CAD build for the part. Positions are in the model's coordinates, mm. A direction names the side the tool comes from. Coordinates: 2 decimals unless noted, no trailing zeros. Loops run counter-clockwise (first coordinate to the right, second up) from the corner with the lowest first, then second, coordinate; pieces in that order, holes last. Notation, with made-up numbers: (88.5, 13.5) -> (134.5, 13.5) arc R30 ccw to (134.5, 52.5) -> close; hole circle Ø10 at (-19.75, 32.5). An arc over 180 degrees is marked (long way). Answer as CSV lines item,"result". Start each with the question number.
from build123d import *

# Parameters (mm, degrees)
SKETCH2_W           = 120
SKETCH2_H           = 55
BOSS_EXTRUDE1_DEPTH = 20
SKETCH3_W           = 20
SKETCH3_H           = 35
CUT_EXTRUDE1_DEPTH  = 20
BOSS_EXTRUDE2_DEPTH = 10


with BuildPart() as part:
    # Sketch2 → Boss-Extrude1 (new body)
    with BuildSketch(Plane(origin=(0, 0, 0), x_dir=(1, 0, 0), z_dir=(0, 1, 0))):
        Rectangle(SKETCH2_W, SKETCH2_H)
    extrude(amount=BOSS_EXTRUDE1_DEPTH)

    # Sketch3 → Cut-Extrude1 (cut)
    with BuildSketch(Plane(origin=(0, 0, 0), x_dir=(-1, 0, 0), z_dir=(0, -1, 0))):
        with Locations((40, 0)):
            Rectangle(SKETCH3_W, SKETCH3_H)
        with Locations((-40, 0)):
            Rectangle(SKETCH3_W, SKETCH3_H)
    extrude(amount=-CUT_EXTRUDE1_DEPTH, mode=Mode.SUBTRACT)

    # Sketch4 → Boss-Extrude2 (add)
    with BuildSketch(Plane(origin=(0, 20, 0), x_dir=(1, 0, 0), z_dir=(0, 1, 0))):
        with BuildLine():
            ThreePointArc((-60, 27.5), (-87.5, 0), (-60, -27.5))
            Line((-60, -27.5), (-60, 27.5))
        make_face()
        with BuildLine():
            ThreePointArc((60, 27.5), (87.5, 0), (60, -27.5))
            Line((60, -27.5), (60, 27.5))
        make_face()
    extrude(amount=-BOSS_EXTRUDE2_DEPTH)


solid = part.part
Item 1: Which spindle directions (+Z, -Z, +X, -X, +Y, -Y) get a long thin tool onto all of the face, cutting with end or side? Do faces 5 (the face through (-71, 10, 0)), 6 (the face through (-87.493, 15.07, -0.605)), 7 (the face through (40, 10, 17.5)), 8 (the face through (71, 10, 0)). Say none if no direction does.
Item 2: Saw through at D-D (y = 12.5). Write the cut outline in (x, z), plus the area to 3 significant figures.
Item 3: Saw through at B-B (y = 5.5). Write the cut outline in (x, z).
Item 4: Saw through at C-C (z = -6.5). Write the cut outline in (x, y), plus the area to 3 significant figures.
Item 5: Flat gauge pins, fed straight in: pin 1 Ø10 at (y, z) = (16, 19) entering from +X; pin 2 Ø12 at (y, z) = (3, 1.5) entering from +X; pin 3 Ø6 at (y, z) = (13.5, 3) entering from -X. Where does each tip first touch, or does it go through?
Item 6: Wall check: probe 1 along X at (y, z) = (2.25, -3.5); probe 2 along Z at (x, y) = (36, 15.5); probe 3 along X at (y, z) = (14.5, -14.5). Give the ranges that are in metal, low to high.
Item 7: Two-plate mould, pull along Z, no slides. Class faces 1 (the face through (87.493, 15.07, -0.605)), 2 (the face through (50, 10, 0)), 3 (the face through (40, 10, -17.5)), 4 (the face through (60, 5, 0)): pulls with the +Z half, pulls with the -Z half, needs draft (parallel to the pull), parting line crosses it, or undercut.
Item 8: Saw through at A-A (z = 0). Write the cut outline in (x, y).
Geometry check:
1,face 5,"+Z, -Z, -X, -Y"
1,face 6,"-X, +Y, -Y"
1,face 7,"+Y, -Y"
1,face 8,"+Z, -Z, +X, -Y"
2,outline,"(-60, -27.5) -> (60, -27.5) arc R27.5 ccw to (60, 27.5) -> (-60, 27.5) arc R27.5 ccw to start; hole (-50, -17.5) -> (-30, -17.5) -> (-30, 17.5) -> (-50, 17.5) -> close; hole (30, -17.5) -> (50, -17.5) -> (50, 17.5) -> (30, 17.5) -> close"
2,area,"7,580 mm2"
3,outline,"(-60, -27.5) -> (60, -27.5) -> (60, 27.5) -> (-60, 27.5) -> close; hole (-50, -17.5) -> (-30, -17.5) -> (-30, 17.5) -> (-50, 17.5) -> close; hole (30, -17.5) -> (50, -17.5) -> (50, 17.5) -> (30, 17.5) -> close"
4,outline,"(-86.72, 10) -> (-60, 10) -> (-60, 0) -> (-50, 0) -> (-50, 20) -> (-86.72, 20) -> close; (-30, 0) -> (30, 0) -> (30, 20) -> (-30, 20) -> close; (50, 0) -> (60, 0) -> (60, 10) -> (86.72, 10) -> (86.72, 20) -> (50, 20) -> close"
4,area,"2,130 mm2"
5,pin 1,"x = 83.67"
5,pin 2,"x = 60"
5,pin 3,"x = -87.5"
6,probe 1,"-60 to -50, -30 to 30, 50 to 60"
6,probe 2,"-27.5 to -17.5, 17.5 to 27.5"
6,probe 3,"-83.37 to -50, -30 to 30, 50 to 83.37"
7,face 1,"parting line crosses it"
7,face 2,"undercut"
7,face 3,"undercut"
7,face 4,"needs draft"
8,outline,"(-87.5, 10) -> (-60, 10) -> (-60, 0) -> (-50, 0) -> (-50, 20) -> (-87.5, 20) -> close; (-30, 0) -> (30, 0) -> (30, 20) -> (-30, 20) -> close; (50, 0) -> (60, 0) -> (60, 10) -> (87.5, 10) -> (87.5, 20) -> (50, 20) -> close"
